```python
from build123d import *

# Parameters (mm, degrees)
BASPROSKE_W        = 5
BASPROSKE_H        = 11
TOOTHCUT_DEPTH     = 17.340134638
TEETHCUTS_COUNT    = 20
TEETHCUTS_ANGLE    = 342
BORSKE_R           = 2.5
BORE_DEPTH         = 50.0000508
SKETCH1_R          = 0.9
CUT_EXTRUDE1_DEPTH = 10


with BuildPart() as part:
    # BasProSke → Base-Revolve (revolve)
    with BuildSketch(Plane(origin=(0, 0, 0), x_dir=(1, 0, 0), z_dir=(0, 1, 0)), mode=Mode.PRIVATE) as base_revolve_sk:
        with Locations((2.5, 5.5)):
            Rectangle(BASPROSKE_W, BASPROSKE_H)
    revolve(base_revolve_sk.sketch.rotate(Axis((-10, 0, 0), (1, 0, 0)), 180), axis=Axis((-10, 0, 0), (1, 0, 0)))

    # TooCutSke → ToothCut (cut, through all)
    with BuildSketch(Plane(origin=(0, 0, 0), x_dir=(0, 0, -1), z_dir=(1, 0, 0))):
        with BuildLine():
            ThreePointArc((0.499924007, 8.734705318), (0, 8.749), (-0.499924007, 8.734705318))
            ThreePointArc((-0.499924007, 8.734705318), (-0.824302243, 9.905497836), (-1.485192705, 10.924909509))
            ThreePointArc((-1.485192705, 10.924909509), (0, 11.0254), (1.485192705, 10.924909509))
            ThreePointArc((1.485192705, 10.924909509), (0.824302243, 9.905497836), (0.499924007, 8.734705318))
        make_face()
    toothcut = extrude(amount=TOOTHCUT_DEPTH, mode=Mode.SUBTRACT)

    # TeethCuts: ToothCut ×20 about axis
    teethcuts_axis = Axis((-10, 0, 0), (1, 0, 0))
    for i in range(1, TEETHCUTS_COUNT):
        add(toothcut.rotate(teethcuts_axis, i * TEETHCUTS_ANGLE / (TEETHCUTS_COUNT - 1)), mode=Mode.SUBTRACT)

    # BorSke → Bore (cut, symmetric)
    with BuildSketch(Plane(origin=(0, 0, 0), x_dir=(0, 0, -1), z_dir=(1, 0, 0))):
        with Locations(Location((0, 0, 0), (0, 0, 180))):
            Circle(BORSKE_R)
    extrude(amount=BORE_DEPTH, both=True, mode=Mode.SUBTRACT)

    # Sketch1 → Cut-Extrude1 (cut)
    with BuildSketch(Plane(origin=(5, 0, 0), x_dir=(0, 0, -1), z_dir=(1, 0, 0))):
        with Locations((6, 0)):
            Circle(SKETCH1_R)
        with Locations((-6, 0)):
            Circle(SKETCH1_R)
    extrude(amount=-CUT_EXTRUDE1_DEPTH, mode=Mode.SUBTRACT)


solid = part.part
```
Geometry check sheet. Reference: the model listing, model coordinates, mm. A direction names the side the tool comes from. Coordinates: 2 decimals unless noted, no trailing zeros. Order: outer loops, then holes, each group sorted by start corner. A loop starts at its lowest first (then second) coordinate and runs counter-clockwise, first axis right, second up.
Q1. Sectioned sample at A-A on z = 0. Record the cut outline in (x, y), and give its area (3 significant figures).
Reply:
outline: (0, -8.75) - (5, -8.75) - (5, -2.5) - (0, -2.5) - close; (0, 2.5) - (5, 2.5) - (5, 8.75) - (0, 8.75) - close
area: 62.5 mm2
Q2. Sectioned sample at B-B on y = 0. Record the cut outline in (x, z).
Reply:
outline: (0, -8.75) - (5, -8.75) - (5, -6.9) - (0, -6.9) - close; (0, -5.1) - (5, -5.1) - (5, -2.5) - (0, -2.5) - close; (0, 2.5) - (5, 2.5) - (5, 5.1) - (0, 5.1) - close; (0, 6.9) - (5, 6.9) - (5, 8.75) - (0, 8.75) - close
Q3. Sectioned sample at D-D on z = 6. Record the cut outline in (x, y), and give its area (3 significant figures).
Reply:
outline: (0, -7.2) - (5, -7.2) - (5, -0.9) - (0, -0.9) - close; (0, 0.9) - (5, 0.9) - (5, 7.2) - (0, 7.2) - close
area: 63.0 mm2
Q4. Thickness scan on probe 1 along Y at (x, z) = (4.65, 9.75); probe 2 along Y at (x, z) = (1.1, -6); probe 3 along Z at (x, y) = (2.85, 10.25). Record the ranges inside material, lowest first.
Reply:
probe 1: y = -5.09 to -4.51, -2.27 to -0.76, 0.76 to 2.27, 4.51 to 5.09
probe 2: y = -7.2 to -0.9, 0.9 to 7.2
probe 3: z = -2.17 to -1, 1 to 2.17
Q5. Draft check along Y on faces 5 (the face through (2.465, 2.277, -9.677)), 6 (the face through (2.46, 9.17, -3.85)), 7 (the face through (2.465, -7.513, -6.461)). Enter one of: released by +Y, released by -Y, zero draft, split by the parting line, or undercut.
Reply:
face 5: undercut
face 6: released by +Y
face 7: released by -Y
Q6. Depth check by flat-ended pin: pin 1 Ø1.6 at (y, z) = (0, -6) entering from +X; pin 2 Ø2 at (x, z) = (1.5, 7.5) entering from +Y; pin 3 Ø2 at (x, y) = (1, -4.5) entering from +Z; pin 4 Ø1.5 at (x, z) = (3.5, 6.5) entering from -Y. Enter the tip coordinate at first touch or a pass-through.
Reply:
pin 1: passes through
pin 2: stops at y = 7.96
pin 3: stops at z = 9.92
pin 4: stops at y = -7.86
Q7. Sectioned sample at C-C on x = 2.9. Give the number of separate pieces and of enclosed holes in the cut face, and give its area (3 significant figures).
Reply:
separate pieces: 1
enclosed holes: 3
area: 278 mm2
Q8. Tool access check on faces 1 (the face through (2.46, 9.64, -2.28)), 2 (the face through (2.465, 9.876, 0.811)), 3 (the face through (2.465, -0.811, 9.876)), 4 (the face through (2.46, 3.82, -9.14)). Record the directions out of +Z, -Z, +X, -X, +Y, -Y that give a thin tool (end or side, any length) a straight path to the whole face; none if there is none.
Reply:
face 1: +X, -X
face 2: +X, -X, +Y
face 3: +Z, +X, -X
face 4: -Z, +X, -X
